from build123d import *

# Parameters (mm, degrees)
BOSS_EXTRUDE1_DEPTH = 6


with BuildPart() as part:
    # Sketch1 → Boss-Extrude1 (new body)
    with BuildSketch(Plane.XY):
        with BuildLine():
            ThreePointArc((483.92628469, -13.296951286), (489.42628469, -7.796951286), (483.92628469, -2.296951286))
            Line((483.92628469, -2.296951286), (0.214631564, 6.146253598))
            Line((0.214631564, 6.146253598), (0, 6.15))
            ThreePointArc((0, 6.15), (-6.15, 0), (0, -6.15))
            Line((0, -6.15), (483.763864662, -13.294552557))
            Line((483.763864662, -13.294552557), (483.92628469, -13.296951286))
        make_face()
        with BuildLine():
            ThreePointArc((0, -5.15), (-5.15, 0), (0, 5.15))
            ThreePointArc((0, 5.15), (0.08987975, 5.149215633), (0.179732122, 5.146862769))
            Line((0.179732122, 5.146862769), (483.92628469, -3.296951286))
            ThreePointArc((483.92628469, -3.296951286), (488.42628469, -7.796951286), (483.92628469, -12.296951286))
            Line((483.92628469, -12.296951286), (0, -5.15))
        make_face(mode=Mode.SUBTRACT)
    extrude(amount=BOSS_EXTRUDE1_DEPTH)


solid = part.part
The model under review builds one solid part; all positions refer to its coordinate system, in mm. Coordinates: 2 decimals unless noted, no trailing zeros. Write each loop counter-clockwise with the first axis right and the second up, starting at its lowest first coordinate (ties: lowest second). Pieces come first, ordered by that corner, then holes. Notation, with made-up numbers: (21.25, -14) -> (30.25, -14) arc R33 cw to (30.25, 24) -> close; hole circle Ø7 at (71, 13.25). An arc over 180 degrees is marked (long way). Answer in a Markdown table with one row per item.
1. Wall thickness on probe 1 along Y at (x, z) = (453, 2.25); probe 2 along Y at (x, z) = (151, 0.7); probe 3 along X at (y, z) = (-4.75, 5.15): over which ranges is each line inside the solid? List them lowest first. Write a range as [from, to].
Answers below:
| item | result |
|---|---|
| probe 1 | y = [-12.84, -11.84], [-2.76, -1.76] |
| probe 2 | y = [-8.38, -7.38], [2.51, 3.51] |
| probe 3 | x = [-3.91, -1.99], [487.24, 488.51] |
2. Clearance check with flat-ended pins moving along their axes: pin 1 Ø1 at (x, y) = (398.5, -4) entering from -Z; pin 2 Ø1 at (x, z) = (335, 1.5) entering from +Y; pin 3 Ø3 at (x, y) = (132.5, -9.5) entering from +Z. State where each tip first meets the part, or that it passes through.
Answers below:
| item | result |
|---|---|
| pin 1 | passes through |
| pin 2 | stops at y = 0.31 |
| pin 3 | stops at z = 6 |
3. We need section A-A, the plane z = 4.7. State the section outline as (x, y) points, and give its area (3 significant figures).
Answers below:
| item | result |
|---|---|
| outline | (0, -6.15) -> (483.93, -13.3) arc R5.5 ccw to (483.93, -2.3) -> (0, 6.15) arc R6.15 ccw to start; hole (0, -5.15) -> (483.93, -12.3) arc R4.5 ccw to (483.93, -3.3) -> (0.18, 5.15) arc R5.15 ccw to (0, 5.15) arc R5.15 ccw to start |
| area | 1,000 mm^2 |
4. We need section B-B, the plane x = 270. State the section outline as (y, z) points.
Answers below:
| item | result |
|---|---|
| outline | (-10.14, 0) -> (-9.14, 0) -> (-9.14, 6) -> (-10.14, 6) -> close; (0.44, 0) -> (1.44, 0) -> (1.44, 6) -> (0.44, 6) -> close |
